Read the model definition and answer for the solid it produces. Units are mm, in the model's axes. Coordinates: 2 decimals unless noted, no trailing zeros. Loops run counter-clockwise (first coordinate to the right, second up) from the corner with the lowest first, then second, coordinate; pieces in that order, holes last. Notation, with made-up numbers: (53, 23.5) - (91, 23.5) arc R27 cw to (91, 62.5) - close; hole circle Ø9 at (-18.5, -13). An arc over 180 degrees is marked (long way). Use one line per item in the form item = value.
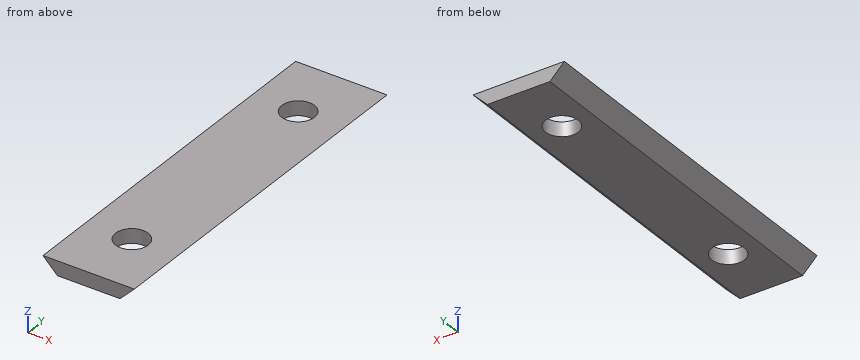
Autodesk Fusion 360 part; units mm, degrees
sketch "Sketch1" plane through (0, 0, 0) normal (0, 1, 0) x (1, 0, 0)
  line L0 (-3.25, 0) -> (3.25, 0)
  line L1 (-4.75, -1.5) -> (4.75, -1.5)
  line L2 (0, -1.5) -> (0, 0) construction
  line L3 (-3.25, 0) -> (-4.75, -1.5)
  line L4 (3.25, 0) -> (4.75, -1.5)
  dimension "d1" = 6.5
  dimension "d2" = 9.5
  dimension "d3" = 45
extrude "Extrude1" add sketch "Sketch1" along normal blind 38
sketch "Sketch2" plane through (0, 0, 1.5) normal (0, 0, 1) x (-1, 0, 0)
  line L0 (4.75, 0) -> (-4.75, 0)
  line L1 (-4.75, 0) -> (-4.75, -38)
  line L2 (-4.75, -38) -> (4.75, -38)
  line L3 (4.75, -38) -> (4.75, 0)
  line L4 (0, 0) -> (0, -38) construction
  point P0 (0, -31.5)
  point P1 (0, -6.5)
  dimension "d6" = 25
  dimension "d7" = 6.5
hole "Hole1" at (0, 31.5, 1.5) at (0, 6.5, 1.5) direction (0, 0, -1) diameter 3.4 depth 16 tip angle 118
Item 1: The part is cut by section D-D on y = 17. Give the vertices of the cut face in (x, z), plus the area to 3 significant figures.
Results below:
outline = (-4.75, 1.5) - (-3.25, 0) - (3.25, 0) - (4.75, 1.5) - close
area = 12.0 mm²
Item 2: The part is cut by section B-B on x = 0. Give the vertices of the cut face in (y, z), plus the area to 3 significant figures.
Results below:
outline = (0, 0) - (4.8, 0) - (4.8, 1.5) - (0, 1.5) - close; (8.2, 0) - (29.8, 0) - (29.8, 1.5) - (8.2, 1.5) - close; (33.2, 0) - (38, 0) - (38, 1.5) - (33.2, 1.5) - close
area = 46.8 mm²
Item 3: Find the intervals of material crossed by L1, parallel to Y at x = 0, z = 1.15; L2, parallel to X at y = 6.5, z = 1.1; L3, parallel to Y at x = 0.75, z = 0.5, in increasing order.
Results below:
L1 = 0 to 4.8, 8.2 to 29.8, 33.2 to 38
L2 = -4.35 to -1.7, 1.7 to 4.35
L3 = 0 to 4.97, 8.03 to 29.97, 33.03 to 38
Item 4: The part is cut by section A-A on y = 6.5. Give the vertices of the cut face in (x, z), plus the area to 3 significant figures.
Results below:
outline = (-4.75, 1.5) - (-3.25, 0) - (-1.7, 0) - (-1.7, 1.5) - close; (1.7, 0) - (3.25, 0) - (4.75, 1.5) - (1.7, 1.5) - close
area = 6.90 mm²
Item 5: The part is cut by section C-C on z = 1.2. Give the vertices of the cut face in (x, y).
Results below:
outline = (-4.45, 0) - (4.45, 0) - (4.45, 38) - (-4.45, 38) - close; hole circle Ø3.4 at (0, 6.5); hole circle Ø3.4 at (0, 31.5)
